from build123d import *

# Parameters (mm, degrees)
PAD113_DEPTH    = 3
PAD114_DEPTH    = 20
SKETCH279_R     = 2
POCKET134_DEPTH = 3.001


with BuildPart() as part:
    # Sketch277 → Pad113 (new body)
    with BuildSketch(Plane.XY):
        with BuildLine():
            ThreePointArc((71.205245, 39.64925), (48.53257, 65.473961), (17.230996, 79.65766))
            ThreePointArc((17.230996, 79.65766), (10.402187, 79.600128), (16.596726, 76.725476))
            ThreePointArc((68.584193, 38.189769), (46.746095, 63.063877), (16.596726, 76.725476))
            ThreePointArc((68.584193, 38.189769), (73.135876, 33.098784), (71.205245, 39.64925))
        make_face()
    extrude(amount=PAD113_DEPTH)

    # Sketch278 (on Face6 of Pad113) → Pad114 (join)
    with BuildSketch(Plane.XY.offset(3)):
        with BuildLine():
            ThreePointArc((66.549812, 41.633791), (46.746095, 63.063877), (20.483489, 75.78045))
            Line((20.483489, 75.78045), (21.266298, 78.676519))
            ThreePointArc((69.093116, 43.224892), (48.53257, 65.473961), (21.266298, 78.676519))
            Line((66.549812, 41.633791), (69.093116, 43.224892))
        make_face()
    extrude(amount=PAD114_DEPTH)

    # Sketch279 (on Face5 of Pad114) → Pocket134 (cut, through all)
    with BuildSketch(Plane.XY.offset(3)):
        with Locations((71.402069, 36.060539)):
            Circle(SKETCH279_R)
        with Locations((14.00263, 79.004593)):
            Circle(SKETCH279_R)
    extrude(amount=-POCKET134_DEPTH, mode=Mode.SUBTRACT)


with BuildPart() as part_1:
    # Body099 placement: moved
    add(part.part.moved(Location((0, 0, 10))))


solid = part_1.part
Design review of the part built by this model. Coordinates are the model's own, in mm. A direction names the side the tool comes from. Round coordinates to 2 decimals unless told otherwise and drop trailing zeros. Loops run counter-clockwise (first coordinate to the right, second up) from the corner with the lowest first, then second, coordinate; pieces in that order, holes last. Notation, with made-up numbers: (-27.75, 33) -> (3.25, 33) arc R22 ccw to (3.25, 49) -> close; hole circle Ø1 at (52, 62.25). An arc over 180 degrees is marked (long way). Use one line per item in the form item = value. Start each with the question number.
Q1. Draft analysis for pull direction X (two halves, no side actions). For faces 3 (the face through (13.57, 77.05, 11.52)), 4 (the face through (20.87, 77.21, 22.86)), 5 (the face through (16, 77, 13)), state which applies: +X half, -X half, draft (parallel to the pull), parting line (faces both ways), or undercut.
Q2. We need section A-A on y = 69.5. Give the boundary of the cut face in (x, z), then the cut area to 3 significant figures.
Q3. We need section B-B on x = 40.5. Give the boundary of the cut face in (y, z).
Q4. We need section C-C on z = 15.25. Give the boundary of the cut face in (x, y), then the cut area to 3 significant figures.
Q5. Wall thickness on line 1 along X through (y, z) = (59.5, 23); line 2 along Y through (x, z) = (26, 31.5); line 3 along Y through (x, z) = (40, 17.25): over which ranges is each line inside the solid? List them lowest first. Write a range as [from, to].
Q6. Machinability: for faces 1 (the face through (47, 64, 33)), 2 (the face through (67.804, 42.418, 22.86)), which of the approach directions +Z, -Z, +X, -X, +Y, -Y give a long, thin tool a straight path to every point of the face, cutting with its end or side? Answer none if there is none.
Q7. For pin 1 Ø4 at (x, z) = (28, 24.5) entering from -Y; pin 2 Ø4 at (y, z) = (70, 28) entering from -X; pin 3 Ø12 at (x, z) = (32, 28) entering from +Y; pin 4 Ø3 at (x, y) = (14, 79) entering from -Z, all flat-tipped, find the tip position at first contact; note any pin that passes through.
Calculated:
q1.face_3 = undercut
q1.face_4 = -X half
q1.face_5 = draft
q2.outline = (36.5, 10) -> (42.57, 10) -> (42.57, 33) -> (36.5, 33) -> close
q2.area = 140 mm²
q3.outline = (67.25, 10) -> (70.72, 10) -> (70.72, 33) -> (67.25, 33) -> close
q4.outline = (20.48, 75.78) arc R78.5 cw to (66.55, 41.63) -> (69.09, 43.22) arc R81.5 ccw to (21.27, 78.68) -> close
q4.area = 179 mm²
q5.line_1 = [51.21, 55.7]
q5.line_2 = [74.07, 77.24]
q5.line_3 = [67.54, 71.01]
q6.face_1 = +Z, +X, -X, +Y, -Y
q6.face_2 = +Z, +X, -Y
q7.pin_1 = 72.54
q7.pin_2 = 31.28
q7.pin_3 = 77.24
q7.pin_4 = through
